Read the model definition and answer for the solid it produces. Units are mm, in the model's axes. A direction names the side the tool comes from. Give positions to 0.01 mm unless a question says otherwise; leave off trailing zeros. Write each loop counter-clockwise with the first axis right and the second up, starting at its lowest first coordinate (ties: lowest second). Pieces come first, ordered by that corner, then holes.
```python
from build123d import *

# Parameters (mm, degrees)
F0_R     = 2.335
F1_DEPTH = 20
F2_R     = 3.125
F3_DEPTH = 4
F4_W     = 1
F4_H     = 1.443127
F6_R     = 1.54834
F7_DEPTH = 5


with BuildPart() as f1:
    # F0 (on Right) → F1 (new body)
    with BuildSketch(Plane.YZ):
        Circle(F0_R)
    extrude(amount=F1_DEPTH)

    # F2 (on face) → F3 (join)
    with BuildSketch(Plane(origin=(0, 0, 0), x_dir=(0, -1, 0), z_dir=(-1, 0, 0))):
        Circle(F2_R)
    extrude(amount=F3_DEPTH)

    # F4 (on Front) → F5 (revolve, cut)
    with BuildSketch(Plane.XZ):
        with BuildLine():
            Line((-1.499683, 3), (-2.499683, 3))
            ThreePointArc((-2.499683, 3), (-1.999683, 2.5), (-1.499683, 3))
        make_face()
        with Locations((-1.999683, 3.721563)):
            Rectangle(F4_W, F4_H)
    revolve(axis=Axis((-1.744851, 0, 0), (1, 0, 0)), mode=Mode.SUBTRACT)

    # F6 (on face) → F7 (cut)
    with BuildSketch(Plane.YZ.offset(20)):
        Circle(F6_R)
    extrude(amount=-F7_DEPTH, mode=Mode.SUBTRACT)


solid = f1.part
```
Item 1: Which of the six approach directions +Z, -Z, +X, -X, +Y, -Y give full straight-line access (tool end or side, diameter ignored) to faces 4 (the flat face through (20, 0, -2)), 5 (the cylindrical face through (9.86, -1.853, -1.421))?
Result set:
face 4: +Z, -Z, +X, +Y, -Y
face 5: +X
Item 2: This flat-tipped pin is pushed along its axis until it touches: pin 1 Ø3 at (x, z) = (17, 1.5) entering from -Y (3 decimals). Where does it stop, or does it pass through?
Result set:
pin 1: stops at y = -2.335
Item 3: Determine the mould class of faces 1 (the flat face through (-4, 0, 0)), 2 (the cylindrical face through (17.54, -1.23, -0.94)), 3 (the cylindrical face through (-3.24, -2.98, 0.94)) for opening direction Y: pulls with the +Y half, pulls with the -Y half, needs draft (parallel to the pull), parting line crosses it, or undercut.
Result set:
face 1: needs draft
face 2: undercut
face 3: parting line crosses it
Item 4: Find the intervals of material crossed by line 1 along Z through (x, y) = (18.5, 0) (3 decimals); line 2 along Z through (x, y) = (4.5, 0) (3 decimals); line 3 along X through (y, z) = (1, -1), in increasing order.
Result set:
line 1: z = -2.335 to -1.548, 1.548 to 2.335
line 2: z = -2.335 to 2.335
line 3: x = -4 to 15
Item 5: Section C-C (x = 4) is taken. Write down the section's boundary in (y, z) (3 decimals), and give its area (3 significant figures).
Result set:
outline: circle Ø4.67 at (0, 0)
area: 17.1 mm2
Item 6: Section A-A (z = 0) is taken. Write down the section's boundary in (x, y) (3 decimals), and give its area (3 significant figures).
Result set:
outline: (-4, -3.125) - (-2.5, -3.125) - (-2.5, -3) arc R0.5 cw to (-1.5, -3) - (-1.5, -3.125) - (0, -3.125) - (0, -2.335) - (20, -2.335) - (20, -1.548) - (15, -1.548) - (15, 1.548) - (20, 1.548) - (20, 2.335) - (0, 2.335) - (0, 3.125) - (-1.5, 3.125) - (-1.5, 3) arc R0.5 cw to (-2.5, 3) - (-2.5, 3.125) - (-4, 3.125) - close
area: 102 mm2
